Design review of the part built by this model. Coordinates are the model's own, in mm. A direction names the side the tool comes from. Round coordinates to 2 decimals unless told otherwise and drop trailing zeros. Loops run counter-clockwise (first coordinate to the right, second up) from the corner with the lowest first, then second, coordinate; pieces in that order, holes last. Notation, with made-up numbers: M -38,4 L -31,4 A18 ccw -31,29 Z; hole C -21.75,67.25 d6. An arc over 180 degrees is marked long. Answer as CSV lines item,"result". Start each with the question number.
from build123d import *

# Parameters (mm, degrees)
SKETCH_1_R          = 1.5
EXTRUDE_1_DEPTH     = 1.5
SKETCH_2_W          = 40
SKETCH_2_H          = 1.5
EXTRUDE_2_DEPTH     = 40
SKETCH_3_R          = 1.75
CUT_EXTRUDE_1_DEPTH = 40
FILLET_1_R          = 3
FILLET_2_R          = 1


with BuildPart() as part:
    # 草图1 → 凸台-拉伸1 (new body)
    with BuildSketch(Plane.XY):
        with BuildLine():
            Line((-20, 0), (-20, -26))
            Line((-20, -26), (20, -26))
            Line((20, -26), (20, 0))
            ThreePointArc((20, 0), (0, 20), (-20, 0))
        make_face()
        with Locations((-7.75, 13.423393759)):
            Circle(SKETCH_1_R, mode=Mode.SUBTRACT)
        with Locations((7.75, 13.423393759)):
            Circle(SKETCH_1_R, mode=Mode.SUBTRACT)
        with Locations((15.5, 0)):
            Circle(SKETCH_1_R, mode=Mode.SUBTRACT)
        with Locations((7.75, -13.423393759)):
            Circle(SKETCH_1_R, mode=Mode.SUBTRACT)
        with Locations((-7.75, -13.423393759)):
            Circle(SKETCH_1_R, mode=Mode.SUBTRACT)
        with Locations((-15.5, 0)):
            Circle(SKETCH_1_R, mode=Mode.SUBTRACT)
        with BuildLine():
            Line((-6.5, 7), (-6.5, -7))
            ThreePointArc((-6.5, -7), (0, -13.5), (6.5, -7))
            Line((6.5, -7), (6.5, 7))
            ThreePointArc((6.5, 7), (0, 13.5), (-6.5, 7))
        make_face(mode=Mode.SUBTRACT)
    extrude(amount=EXTRUDE_1_DEPTH)

    # 草图2 → 凸台-拉伸2 (add)
    with BuildSketch(Plane(origin=(0, 0, 0), x_dir=(-1, 0, 0), z_dir=(0, 0, -1))):
        with Locations((0, -25.25)):
            Rectangle(SKETCH_2_W, SKETCH_2_H)
    extrude(amount=EXTRUDE_2_DEPTH)

    # 草图3 → 切除-拉伸1 (cut)
    with BuildSketch(Plane(origin=(0, -24.5, 0), x_dir=(1, 0, 0), z_dir=(0, 1, 0))):
        with Locations(Location((-15, 32, 0), (0, 0, 270))):
            Circle(SKETCH_3_R)
        with Locations(Location((-15, 8, 0), (0, 0, 270))):
            Circle(SKETCH_3_R)
        with Locations(Location((15, 8, 0), (0, 0, 270))):
            Circle(SKETCH_3_R)
        with Locations(Location((15, 32, 0), (0, 0, 270))):
            Circle(SKETCH_3_R)
    extrude(amount=-CUT_EXTRUDE_1_DEPTH, mode=Mode.SUBTRACT)

    # 圆角1
    fillet_1_edges = [part.edges().sort_by_distance(p)[0] for p in [
        (20, -25.25, -40),
        (-20, -25.25, -40),
    ]]
    fillet(fillet_1_edges, radius=FILLET_1_R)

    # 圆角2
    fillet_2_edges = [part.edges().sort_by_distance(p)[0] for p in [
        (0, -24.5, 0),
        (0, -26, 1.5),
    ]]
    fillet(fillet_2_edges, radius=FILLET_2_R)


solid = part.part
Item 1: Consider section C-C, the plane y = 9. Write out the cut boundary in (x, z).
Item 2: Insertion check: pin 1 Ø4 at (x, z) = (-15, -8) entering from +Y; pin 2 Ø4 at (x, y) = (-10.5, -15.5) entering from -Z; pin 3 Ø5.5 at (x, z) = (-15, -32) entering from -Y. Each pin has a flat end and moves straight along its axis. Give the tip position at first contact, or say it passes through.
Item 3: Tool access review of faces 4 (the face through (6.5, 0, 1)), 5 (the face through (20, -25, -12)), 6 (the face through (9, -6, 0)): name each direction out of +Z, -Z, +X, -X, +Y, -Y from which nothing blocks a thin tool from reaching the whole face with its end or side.
Item 4: Consider section A-A, the plane z = -8. Write out the cut boundary in (x, y), then the cut area to 3 significant figures.
Item 5: Consider section D-D, the plane x = 16. Write out the cut boundary in (y, z).
Item 6: To check wall thickness, follow line 1 (X direction, y = -25.6, z = -8); line 2 (Y direction, x = -7.75, z = 0.9); line 3 (Z direction, x = 10, y = -2). State the ranges of each line that lie inside material, in increasing order.
Item 7: The part is to be moulded in two halves that separate along Z. For faces 1 (the face through (19.14, -25.24, -39.1)), 2 (the face through (-17, 0, 1)), 3 (the face through (16.735, -25.24, -8.228)), say which applies: +Z half, -Z half, draft (parallel to the pull), parting line (faces both ways), or undercut.
Item 8: Consider section B-B, the plane x = 0. Write out the cut boundary in (y, z), then the cut area to 3 significant figures.
Found:
1,outline,"M -17.86,0 L -6.18,0 L -6.18,1.5 L -17.86,1.5 Z; M 6.18,0 L 17.86,0 L 17.86,1.5 L 6.18,1.5 Z"
2,pin 1,"stops at y = -24.5"
2,pin 2,"stops at z = 0"
2,pin 3,"stops at y = -26"
3,face 4,"+Z, -Z"
3,face 5,"+Z, -Z, +X, +Y, -Y"
3,face 6,"-Z, +X, -X, +Y"
4,outline,"M -20,-26 L -16.75,-26 L -16.75,-24.5 L -20,-24.5 Z; M -13.25,-26 L 13.25,-26 L 13.25,-24.5 L -13.25,-24.5 Z; M 16.75,-26 L 20,-26 L 20,-24.5 L 16.75,-24.5 Z"
4,area,"49.5 mm^2"
5,outline,"M -26,-40 L -24.5,-40 L -24.5,-33.44 L -26,-33.44 Z; M -26,-30.56 L -24.5,-30.56 L -24.5,-9.44 L -26,-9.44 Z; M -26,-6.56 L -24.5,-6.56 L -24.5,-1 A1 cw -23.5,0 L -1.41,0 L -1.41,1.5 L -25,1.5 A1 ccw -26,0.5 Z; M 1.41,0 L 12,0 L 12,1.5 L 1.41,1.5 Z"
6,line 1,"x = -20 to -16.75, -13.25 to 13.25, 16.75 to 20"
6,line 2,"y = -25.92 to -14.92, -11.92 to 11.92, 14.92 to 18.44"
6,line 3,"z = 0 to 1.5"
7,face 1,"-Z half"
7,face 2,"draft"
7,face 3,"undercut"
8,outline,"M -26,-40 L -24.5,-40 L -24.5,-1 A1 cw -23.5,0 L -13.5,0 L -13.5,1.5 L -25,1.5 A1 ccw -26,0.5 Z; M 13.5,0 L 20,0 L 20,1.5 L 13.5,1.5 Z"
8,area,"88.5 mm^2"
